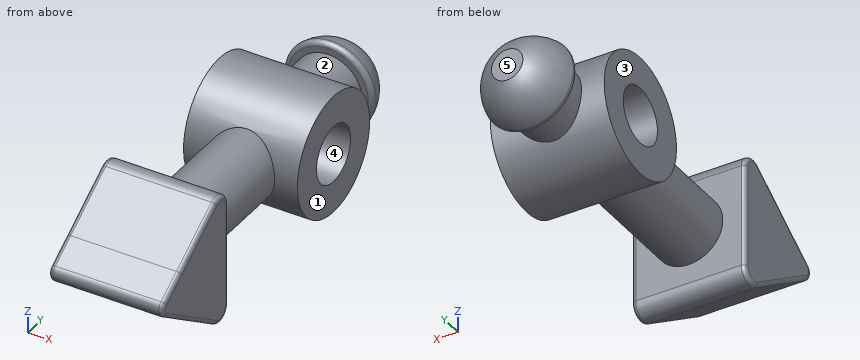
```python
from build123d import *

# Parameters (mm, degrees)
SKETCH1_R                = 16.6116
BOSS_EXTRUDE1_DEPTH      = 31.75
SKETCH5_R                = 7.874
CUT_EXTRUDE4_DEPTH       = 31.75
SKETCH7_R                = 9.525
BOSS_EXTRUDE2_DEPTH      = 14.732
SKETCH8_R                = 12.7
BOSS_EXTRUDE3_DEPTH      = 11.43
FILLET5_R                = 1.27
BOSS_EXTRUDE4_DEPTH      = 15.875
BOSS_EXTRUDE4_DEPTH_BACK = 15.875
BOSS_EXTRUDE5_DEPTH      = 31.75
BOSS_EXTRUDE5_DEPTH_BACK = 3.81
SKETCH13_R               = 9.525
FILLET6_R                = 1.143


with BuildPart() as part:
    # Sketch1 → Boss-Extrude1 (new body)
    with BuildSketch(Plane(origin=(0, 0, 0), x_dir=(0, 0, -1), z_dir=(1, 0, 0))):
        Circle(SKETCH1_R)
    extrude(amount=BOSS_EXTRUDE1_DEPTH)

    # Sketch5 → Cut-Extrude4 (cut)
    with BuildSketch(Plane.ZY):
        Circle(SKETCH5_R)
    extrude(amount=-CUT_EXTRUDE4_DEPTH, mode=Mode.SUBTRACT)

    # Sketch7 → Boss-Extrude2 (add)
    with BuildSketch(Plane(origin=(0, 23.63216, 0), x_dir=(1, 0, 0), z_dir=(0, 1, 0))):
        with Locations(Location((15.875, 0, 0), (0, 0, 270))):
            Circle(SKETCH7_R)
    extrude(amount=-BOSS_EXTRUDE2_DEPTH)

    # Sketch8 → Boss-Extrude3 (add)
    with BuildSketch(Plane(origin=(0, 23.63216, 0), x_dir=(1, 0, 0), z_dir=(0, 1, 0))):
        with Locations(Location((15.875, 0, 0), (0, 0, 270))):
            Circle(SKETCH8_R)
    extrude(amount=BOSS_EXTRUDE3_DEPTH)

    # Sketch10 → Cut-Revolve1 (revolve, cut)
    with BuildSketch(Plane.XY, mode=Mode.PRIVATE) as cut_revolve1_sk:
        with BuildLine():
            Line((11.487410409, 35.062159614), (3.175, 35.06216))
            Line((3.175, 35.06216), (3.175, 23.63216))
            ThreePointArc((3.175, 23.63216), (5.734420744, 30.508413369), (11.487410409, 35.062159614))
        make_face()
    revolve(cut_revolve1_sk.sketch.rotate(Axis((15.875, 35.06216, 0), (0, -1, 0)), 270), axis=Axis((15.875, 35.06216, 0), (0, -1, 0)), mode=Mode.SUBTRACT)

    # Fillet5
    fillet5_edges = [part.edges().sort_by_distance(p)[0] for p in [
        (15.875, 23.63216, -12.7),
    ]]
    fillet(fillet5_edges, radius=FILLET5_R)



with BuildPart() as body_2:
    # Sketch12 → Boss-Extrude4 (new, two sides: drawn at the far end of the back side and taken through both)
    with BuildSketch(Plane(origin=(15.875, 0, 0), x_dir=(0, 0, -1), z_dir=(1, 0, 0)).offset(-BOSS_EXTRUDE4_DEPTH_BACK)):
        with BuildLine():
            Line((2.629138572, -77.398426312), (7.313053442, -70.340553032))
            Line((7.313053442, -70.340553032), (17.972630658, -54.27835991))
            ThreePointArc((17.972630658, -54.27835991), (18.155391887, -50.370302586), (14.798097199, -48.3616))
            Line((14.798097199, -48.3616), (-13.770933928, -48.3616))
            ThreePointArc((-13.770933928, -48.3616), (-17.128181434, -50.370214649), (-16.945577748, -54.278193604))
            Line((-16.945577748, -54.278193604), (-6.287102166, -70.340553032))
            Line((-6.287102166, -70.340553032), (-1.603719855, -77.398426312))
            ThreePointArc((-1.603719855, -77.398426312), (0.512709359, -78.534030576), (2.629138572, -77.398426312))
        make_face()
    extrude(amount=BOSS_EXTRUDE4_DEPTH + BOSS_EXTRUDE4_DEPTH_BACK)


with BuildPart() as part_1:
    add(part.part)

    add(body_2.part)  # Boss-Extrude5 merges body 2
    # Sketch13 → Boss-Extrude5 (add, two sides: drawn at the far end of the back side and taken through both)
    with BuildSketch(Plane(origin=(0, -16.6116, 0), x_dir=(-1, 0, 0), z_dir=(0, -1, 0)).offset(-BOSS_EXTRUDE5_DEPTH_BACK)):
        with Locations(Location((-15.875, 0, 0), (0, 0, 270))):
            Circle(SKETCH13_R)
    extrude(amount=BOSS_EXTRUDE5_DEPTH + BOSS_EXTRUDE5_DEPTH_BACK)

    # Fillet6
    fillet6_edges = [part_1.edges().sort_by_distance(p)[0] for p in [
        (0, -50.370214649, 17.128181434),
        (0, -48.3616, -0.513581636),
        (0, -50.370302586, -18.155391887),
        (0, -65.838393111, -10.300884615),
        (0, -78.534030576, -0.512709359),
        (0, -65.838309958, 9.274648801),
        (31.75, -50.370214649, 17.128181434),
        (31.75, -65.838309958, 9.274648801),
        (31.75, -78.534030576, -0.512709359),
        (31.75, -65.838393111, -10.300884615),
        (31.75, -50.370302586, -18.155391887),
        (31.75, -48.3616, -0.513581636),
    ]]
    fillet(fillet6_edges, radius=FILLET6_R)


solid = part_1.part
```
The model under review builds one solid part; all positions refer to its coordinate system, in mm. Face numbers are marked on the shaded views. A direction names the side the tool comes from. Round coordinates to 2 decimals unless told otherwise and drop trailing zeros. Write each loop counter-clockwise with the first axis right and the second up, starting at its lowest first coordinate (ties: lowest second). Pieces come first, ordered by that corner, then holes. Notation, with made-up numbers: (75, -28.75) - (101, -28.75) arc R31 cw to (101, 5.25) - close; hole circle Ø11 at (84, -4.75). An arc over 180 degrees is marked (long way). Use one line per item in the form item = value.
Q1. Consider section A-A (y = 0). State the section outline as (x, z) points.
Answer key:
outline = (0, -16.61) - (31.75, -16.61) - (31.75, -7.87) - (0, -7.87) - close; (0, 7.87) - (31.75, 7.87) - (31.75, 16.61) - (0, 16.61) - close
Q2. Insertion check: pin 1 Ø10 at (x, y) = (27.5, -63.5) entering from +Z; pin 2 Ø3 at (x, z) = (18, -11.5) entering from -Y; pin 3 Ø3 at (x, y) = (17, -16) entering from +Z (3 decimals). Each pin has a flat end and moves straight along its axis. Give the tip position at first contact, or say it passes through.
Answer key:
pin_1 = 14.14
pin_2 = -66.29
pin_3 = 9.525
Q3. For line 1 (X direction, y = -34, z = -0.5); line 2 (Y direction, x = 25, z = 0); line 3 (Y direction, x = 23, z = -1), list the stretches that pass through material, from the lowest coordinate up. Write a range as [from, to].
Answer key:
line_1 = [6.36, 25.39]
line_2 = [-78.48, -7.87], [7.87, 31.75]
line_3 = [-78.49, -7.81], [7.81, 33.47]
Q4. Draft analysis for pull direction Y (two halves, no side actions). For the marked faces 3, 4 and 5, state which applies: +Y half, -Y half, draft (parallel to the pull), parting line (faces both ways), or undercut.
Answer key:
face_3 = draft
face_4 = undercut
face_5 = +Y half
Q5. Consider section B-B (y = -28). State the section outline as (x, z) points (3 decimals).
Answer key:
outline = circle Ø19.05 at (15.875, 0)
Q6. Tool access review of the marked faces 1 and 2: name each direction out of +Z, -Z, +X, -X, +Y, -Y from which nothing blocks a thin tool from reaching the whole face with its end or side.
Answer key:
face_1 = +Z, -Z, +X, +Y, -Y
face_2 = none
